from build123d import *

# Parameters (mm, degrees)
F0_W     = 104
F0_H     = 5
F0_W_2   = 5
F0_H_2   = 15
F1_DEPTH = 10
F2_DEPTH = 10


with BuildPart() as f1:
    # F0 (on Front) → F1 (new body)
    with BuildSketch(Plane.XZ):
        with Locations((0.4955184162, -87.9514326147)):
            Rectangle(F0_W, F0_H)
        with Locations((-54.0044815838, -87.9514326147)):
            Rectangle(F0_W_2, F0_H)
        with Locations((-54.0044815838, -77.9514326147)):
            Rectangle(F0_W_2, F0_H_2)
        with Locations((54.9955184162, -77.9514326147)):
            Rectangle(F0_W_2, F0_H_2)
        with Locations((54.9955184162, -87.9514326147)):
            Rectangle(F0_W_2, F0_H)
    extrude(amount=F1_DEPTH)

    # F0 (on Front) → F2 (join)
    with BuildSketch(Plane.XZ):
        with Locations((-54.0044815838, -87.9514326147)):
            Rectangle(F0_W_2, F0_H)
        with Locations((54.9955184162, -87.9514326147)):
            Rectangle(F0_W_2, F0_H)
        with Locations((0.4955184162, -87.9514326147)):
            Rectangle(F0_W, F0_H)
        with Locations((-54.0044815838, -77.9514326147)):
            Rectangle(F0_W_2, F0_H_2)
        with Locations((54.9955184162, -77.9514326147)):
            Rectangle(F0_W_2, F0_H_2)
        with Locations((0.4955184162, -77.9514326147)):
            Rectangle(F0_W, F0_H_2)
        Polygon((57.4955184162, 99.5485673853), (-56.5044815838, 99.5485673853), (-56.5044815838, -70.4514326147), (-51.5044815838, -70.4514326147), (52.4955184162, -70.4514326147), (57.4955184162, -70.4514326147), align=None)
    extrude(amount=-F2_DEPTH)


solid = f1.part
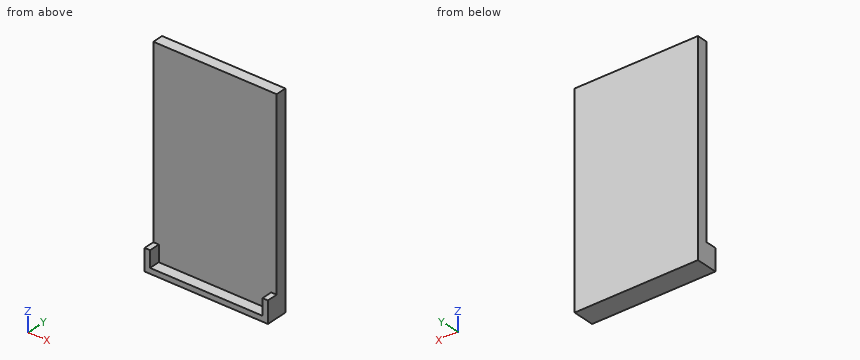
Verification items for the finished model (mm, model axes). Coordinates: 2 decimals unless noted, no trailing zeros. Write each loop counter-clockwise with the first axis right and the second up, starting at its lowest first coordinate (ties: lowest second). Pieces come first, ordered by that corner, then holes. Notation, with made-up numbers: (-30, 16.25) - (-2, 16.25) arc R27 cw to (-2, 48.25) - close; hole circle Ø2 at (29, -21.5). An arc over 180 degrees is marked (long way). Answer as a JSON object with one key per item and string values.
(1) Cross-section at B-B on z = -30. Record the cut outline in (x, y).
Report:
{"outline": "(-56.5, 0) - (57.5, 0) - (57.5, 10) - (-56.5, 10) - close"}
(2) Thickness scan on line 1 along X through (y, z) = (-2.5, -78); line 2 along Y through (x, z) = (16, -20.5); line 3 along Z through (x, y) = (-37, -2). Record the ranges inside material, lowest first.
Report:
{"line 1": "-56.5 to -51.5, 52.5 to 57.5", "line 2": "0 to 10", "line 3": "-90.45 to -85.45"}
(3) Cross-section at A-A on x = 40.5. Record the cut outline in (y, z).
Report:
{"outline": "(-10, -90.45) - (10, -90.45) - (10, 99.55) - (0, 99.55) - (0, -85.45) - (-10, -85.45) - close"}
(4) Gauge pin test, flat ends, axial feed: pin 1 Ø4 at (y, z) = (-0.5, 78.5) entering from +X; pin 2 Ø4 at (x, y) = (55, -5) entering from +Z; pin 3 Ø5 at (x, y) = (19.5, -6.5) entering from +Z. Record the tip position at first contact, or that the pin passes through.
Report:
{"pin 1": "x = 57.5", "pin 2": "z = -70.45", "pin 3": "z = -85.45"}
